Here's how the part is built. I have some questions about the finished solid (model axes, mm). A direction names the side the tool comes from. Round coordinates to 2 decimals unless told otherwise and drop trailing zeros. Order: outer loops, then holes, each group sorted by start corner. A loop starts at its lowest first (then second) coordinate and runs counter-clockwise, first axis right, second up.
```python
from build123d import *

# Parameters (mm, degrees)
F0_W     = 21.635506
F0_H     = 3.251886
F1_DEPTH = 3
F2_DEPTH = 40
F3_W     = 21.635506
F3_H     = 3
F4_DEPTH = 3
F5_R     = 2


with BuildPart() as f1:
    # F0 (on Top) → F1 (new body)
    with BuildSketch(Plane.XY):
        Polygon((71.532905, -23.780284), (71.532905, -23.03217), (71.532905, 20.313235), (60.715152, 20.313235), (49.897399, 20.313235), (49.897399, -23.03217), (49.897399, -23.780284), align=None)
        with BuildLine():
            add(Edge.make_bspline(
                [(60.715152, 16.313235), (60.19191, 16.340598), (60.299679, 16.300383), (59.789945, 15.845333)],
                knots=[0, 0, 0, 0, 1.036794, 1.036794, 1.036794, 1.036794], degree=3))
            add(Edge.make_bspline(
                [(60.715152, 16.313235), (61.238394, 16.340598), (61.130624, 16.300383), (61.640359, 15.845333)],
                knots=[0, 0, 0, 0, 1.036794, 1.036794, 1.036794, 1.036794], degree=3))
            Line((61.640359, 15.845333), (66.269247, 11.295008))
            add(Edge.make_bspline(
                [(66.269247, 11.295008), (67.073074, 10.193584), (67.434184, 9.998059), (67.532905, 8.518658)],
                knots=[0, 0, 0, 0, 3.050401, 3.050401, 3.050401, 3.050401], degree=3))
            Line((67.532905, 8.518658), (67.532905, -11.267474))
            add(Edge.make_bspline(
                [(67.532905, -11.267474), (67.542302, -12.628771), (67.336095, -13.63057), (66.316183, -14.749149)],
                knots=[0, 0, 0, 0, 3.688154, 3.688154, 3.688154, 3.688154], degree=3))
            Line((66.316183, -14.749149), (61.925017, -19.323452))
            add(Edge.make_bspline(
                [(61.925017, -19.323452), (61.584013, -19.632298), (61.069199, -19.584967), (60.715152, -19.595665)],
                knots=[0, 0, 0, 0, 1.240111, 1.240111, 1.240111, 1.240111], degree=3))
            add(Edge.make_bspline(
                [(59.505286, -19.323452), (59.846291, -19.632298), (60.361105, -19.584967), (60.715152, -19.595665)],
                knots=[0, 0, 0, 0, 1.240111, 1.240111, 1.240111, 1.240111], degree=3))
            Line((59.505286, -19.323452), (55.114121, -14.749149))
            add(Edge.make_bspline(
                [(53.897399, -11.267474), (53.888002, -12.628771), (54.094209, -13.63057), (55.114121, -14.749149)],
                knots=[0, 0, 0, 0, 3.688154, 3.688154, 3.688154, 3.688154], degree=3))
            Line((53.897399, -11.267474), (53.897399, 8.518658))
            add(Edge.make_bspline(
                [(55.161057, 11.295008), (54.35723, 10.193584), (53.99612, 9.998059), (53.897399, 8.518658)],
                knots=[0, 0, 0, 0, 3.050401, 3.050401, 3.050401, 3.050401], degree=3))
            Line((55.161057, 11.295008), (59.789945, 15.845333))
        make_face(mode=Mode.SUBTRACT)
        with Locations((60.715152, -25.406227)):
            Rectangle(F0_W, F0_H)
    extrude(amount=F1_DEPTH)

    # F0 (on Top) → F2 (join)
    with BuildSketch(Plane.XY):
        with Locations((60.715152, -25.406227)):
            Rectangle(F0_W, F0_H)
    extrude(amount=F2_DEPTH)

    # F3 (on face) → F4 (join)
    with BuildSketch(Plane.XZ.offset(27.03217)):
        with Locations((60.715152, 38.5)):
            Rectangle(F3_W, F3_H)
    extrude(amount=F4_DEPTH)

    # F5
    f5_edges = [f1.edges().sort_by_distance(p)[0] for p in [
        (60.715152, -30.03217, 40),
        (60.715152, -23.780284, 40),
        (60.715152, -23.780284, 3),
    ]]
    fillet(f5_edges, radius=F5_R)


solid = f1.part
```
1. I need wall thicknesses on probe 1 along Z at (x, y) = (69.5, -19); probe 2 along Y at (x, z) = (57, 23.5); probe 3 along Y at (x, z) = (56.75, 2). Which ranges of each line are inside material? Lowest first, please.
Evaluation:
probe 1: z = 0 to 3
probe 2: y = -27.03 to -23.78
probe 3: y = -27.03 to -16.45, 12.86 to 20.31
2. On a 3-axis mill with a long thin cutter (end or side, diameter ignored), from which of +Z, -Z, +X, -X, +Y, -Y can I reach the whole of each face in a straight line? I mean faces 4 (the flat face through (63.922, 13.602, 1.479)), 5 (the flat face through (68, -3, 0)), 6 (the flat face through (61, -23.78, 21)), 7 (the flat face through (61, -27.032, 18)). Say none if no direction works.
Evaluation:
face 4: +Z, -Z
face 5: -Z, +X, -X, +Y, -Y
face 6: +Z, +X, -X, +Y
face 7: -Z, +X, -X, -Y
3. If we section it at A-A, the plane y = -4: Write out the boundary of the cut face in (x, z), and give its area (3 significant figures).
Evaluation:
outline: (49.9, 0) - (53.9, 0) - (53.9, 3) - (49.9, 3) - close; (67.53, 0) - (71.53, 0) - (71.53, 3) - (67.53, 3) - close
area: 24.0 mm2
4. If we mould it in two halves opening along X, with no side actions, what happens to faces 1 (the flat face through (71.533, -12, 2)), 2 (the flat face through (57.34, -17.07, 1.48)), 3 (the flat face through (61, -27, 40))? For each: released by +X, released by -X, zero draft, split by the parting line, or undercut.
Evaluation:
face 1: released by +X
face 2: undercut
face 3: zero draft
5. If we section it at C-C, the plane z = 12: Write out the boundary of the cut face in (x, y).
Evaluation:
outline: (49.9, -27.03) - (71.53, -27.03) - (71.53, -23.78) - (49.9, -23.78) - close
6. If we section it at B-B, the plane x = 65: Write out the boundary of the cut face in (y, z).
Evaluation:
outline: (-30.03, 37) - (-27.03, 37) - (-27.03, 0) - (-16.12, 0) - (-16.12, 3) - (-21.78, 3) arc R2 cw to (-23.78, 5) - (-23.78, 38) arc R2 ccw to (-25.78, 40) - (-28.03, 40) arc R2 ccw to (-30.03, 38) - close; (12.54, 0) - (20.31, 0) - (20.31, 3) - (12.54, 3) - close
7. If we section it at D-D, the plane y = -21: Write out the boundary of the cut face in (x, z), and give its area (3 significant figures).
Evaluation:
outline: (49.9, 0) - (71.53, 0) - (71.53, 3) - (49.9, 3) - close
area: 64.9 mm2
8. I'm going to push flat-ended pins straight in: P1, Ø6.5, axis at x = 65.5, z = 27, coming from the -Y side; P2, Ø1, axis at x = 52, y = 7, coming from the +Z side. Where does each tip first touch, or does it pass through?
Evaluation:
P1: stops at y = -27.03
P2: stops at z = 3
